Design review of the part built by this model. Coordinates are the model's own, in mm. Coordinates: 2 decimals unless noted, no trailing zeros. Loops run counter-clockwise (first coordinate to the right, second up) from the corner with the lowest first, then second, coordinate; pieces in that order, holes last.
Q1. Wall thickness on probe 1 along Y at (x, z) = (2.25, -25.4); probe 2 along Y at (x, z) = (1.5, 0); probe 3 along Z at (x, y) = (5.75, 3): over which ranges is each line inside the solid? List them lowest first.
Q2. Add section A-A on z = 25.4. Give the boundary of the cut face in (x, y).
Q3. Draft analysis for pull direction Y (two halves, no side actions). For faces 1 (the face through (3.131, -0.099, -27.646)), 2 (the face through (3, -19.05, 0)), 3 (the face through (3, 0, 31.75)), state which applies: released by +Y, released by -Y, zero draft, split by the parting line, or undercut.
Q4. Add section C-C on x = 5.5. Give the boundary of the cut face in (y, z).
Q5. Add section D-D on y = -4. Give the boundary of the cut face in (x, z), and give its area (3 significant figures).
Q6. Add section B-B on y = 0. Give the boundary of the cut face in (x, z).
```python
from build123d import *

# Parameters (mm, degrees)
SKETCH1_W           = 63.5
SKETCH1_H           = 38.1
SKETCH1_R           = 7.2263
SKETCH1_R_2         = 2.2479
BOSS_EXTRUDE1_DEPTH = 6.35


with BuildPart() as part:
    # Sketch1 → Boss-Extrude1 (new body)
    with BuildSketch(Plane(origin=(0, 0, 0), x_dir=(0, 0, -1), z_dir=(1, 0, 0))):
        Rectangle(SKETCH1_W, SKETCH1_H)
        Circle(SKETCH1_R, mode=Mode.SUBTRACT)
        with Locations((-25.4, 0)):
            Circle(SKETCH1_R_2, mode=Mode.SUBTRACT)
        with Locations(Location((25.4, 0, 0), (0, 0, 180))):
            Circle(SKETCH1_R_2, mode=Mode.SUBTRACT)
    extrude(amount=BOSS_EXTRUDE1_DEPTH)


solid = part.part
```
Entries:
1. probe 1: y = -19.05 to -2.25, 2.25 to 19.05
1. probe 2: y = -19.05 to -7.23, 7.23 to 19.05
1. probe 3: z = -31.75 to -6.57, 6.57 to 31.75
2. outline: (0, -19.05) - (6.35, -19.05) - (6.35, -2.25) - (0, -2.25) - close; (0, 2.25) - (6.35, 2.25) - (6.35, 19.05) - (0, 19.05) - close
3. face 1: undercut
3. face 2: released by -Y
3. face 3: zero draft
4. outline: (-19.05, -31.75) - (19.05, -31.75) - (19.05, 31.75) - (-19.05, 31.75) - close; hole circle Ø14.45 at (0, 0); hole circle Ø4.5 at (0, -25.4); hole circle Ø4.5 at (0, 25.4)
5. outline: (0, -31.75) - (6.35, -31.75) - (6.35, -6.02) - (0, -6.02) - close; (0, 6.02) - (6.35, 6.02) - (6.35, 31.75) - (0, 31.75) - close
5. area: 327 mm2
6. outline: (0, -31.75) - (6.35, -31.75) - (6.35, -27.65) - (0, -27.65) - close; (0, -23.15) - (6.35, -23.15) - (6.35, -7.23) - (0, -7.23) - close; (0, 7.23) - (6.35, 7.23) - (6.35, 23.15) - (0, 23.15) - close; (0, 27.65) - (6.35, 27.65) - (6.35, 31.75) - (0, 31.75) - close
